Design review of the part shown in the three views and the two pictorial views. Dimensions are in mm from the part's minimum x, y and z. Give positions to 0.01 mm unless a question says otherwise; leave off trailing zeros. One line per question, with ' | ' between items. Start each with the question number.
(1) Wall thickness on probe 1 along X at (y, z) = (45.5, 2) (1 decimal); probe 2 along Y at (x, z) = (64.5, 4.75) (1 decimal); probe 3 along Y at (x, z) = (60, 1.5) (1 decimal): over which ranges is each line inside the solid? List them lowest first.
(2) Insertion check: P1, Ø4, axis at x = 81.25, y = 47.69, coming from the +Z side; P2, Ø2, axis at x = 31.5, z = 0.5, coming from the -Y side; P3, Ø3, axis at y = 64.5, z = 4.5, coming from the -X side (1 decimal); P4, Ø1.5, axis at y = 17.5, z = 3, coming from the -X side (1 decimal). Each pin has a flat end and moves straight along its axis. Give the tip position at first contact, or say it passes through.
(3) Draft analysis for pull direction Y (two halves, no side actions). For the marked faces 1 and 2, state which applies: +Y half, -Y half, draft (parallel to the pull), parting line (faces both ways), or undercut.
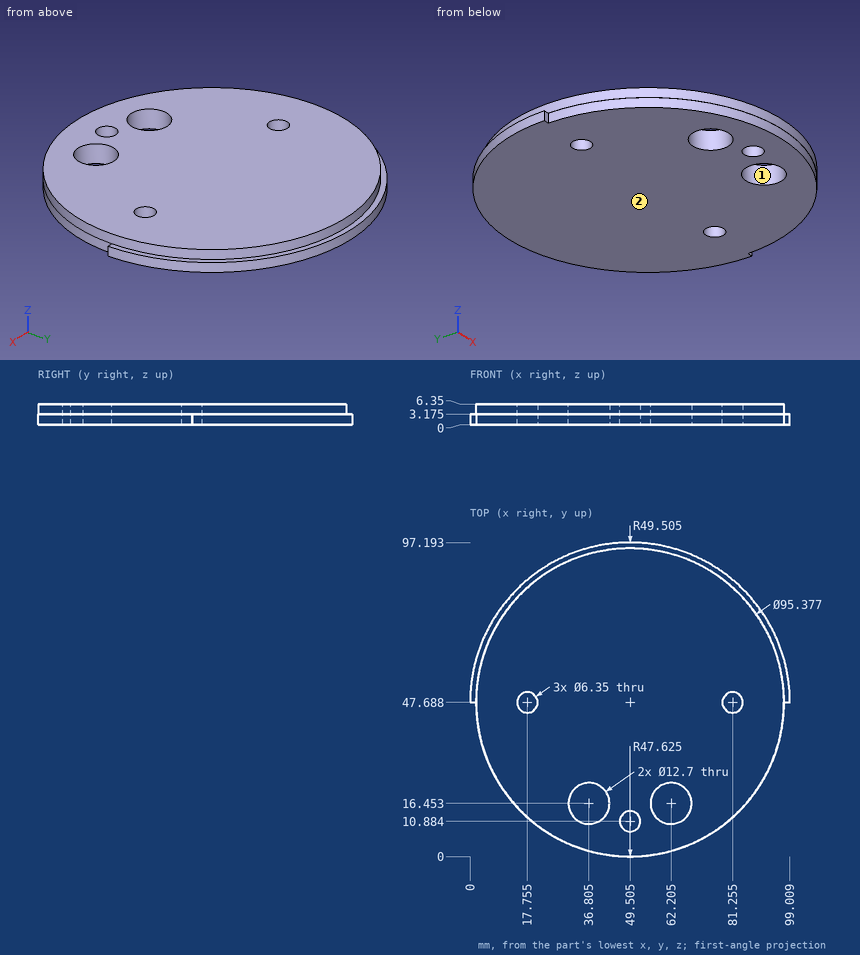
A:
1) probe 1: x = 1.9 to 15.5, 20.1 to 79, 83.6 to 97.1 | probe 2: y = 2.4 to 10.5, 22.4 to 93 | probe 3: y = 1.2 to 10.5, 22.4 to 96.1
2) P1: passes through | P2: stops at y = 3.2 | P3: stops at x = 2.7 | P4: stops at x = 12
3) face 1: undercut | face 2: draft
